Here's the drawing with two shaded views (mm, measured from the low corner). I have some questions. Give positions to 0.01 mm unless a question says otherwise; leave off trailing zeros. Write each loop counter-clockwise with the first axis right and the second up, starting at its lowest first coordinate (ties: lowest second). Pieces come first, ordered by that corner, then holes. Notation, with made-up numbers: (88, -32.75) -> (94, -32.75) arc R19 cw to (94, -22.75) -> close; hole circle Ø9 at (1.5, -38.5). An arc over 180 degrees is marked (long way). One line per item, written item: value.
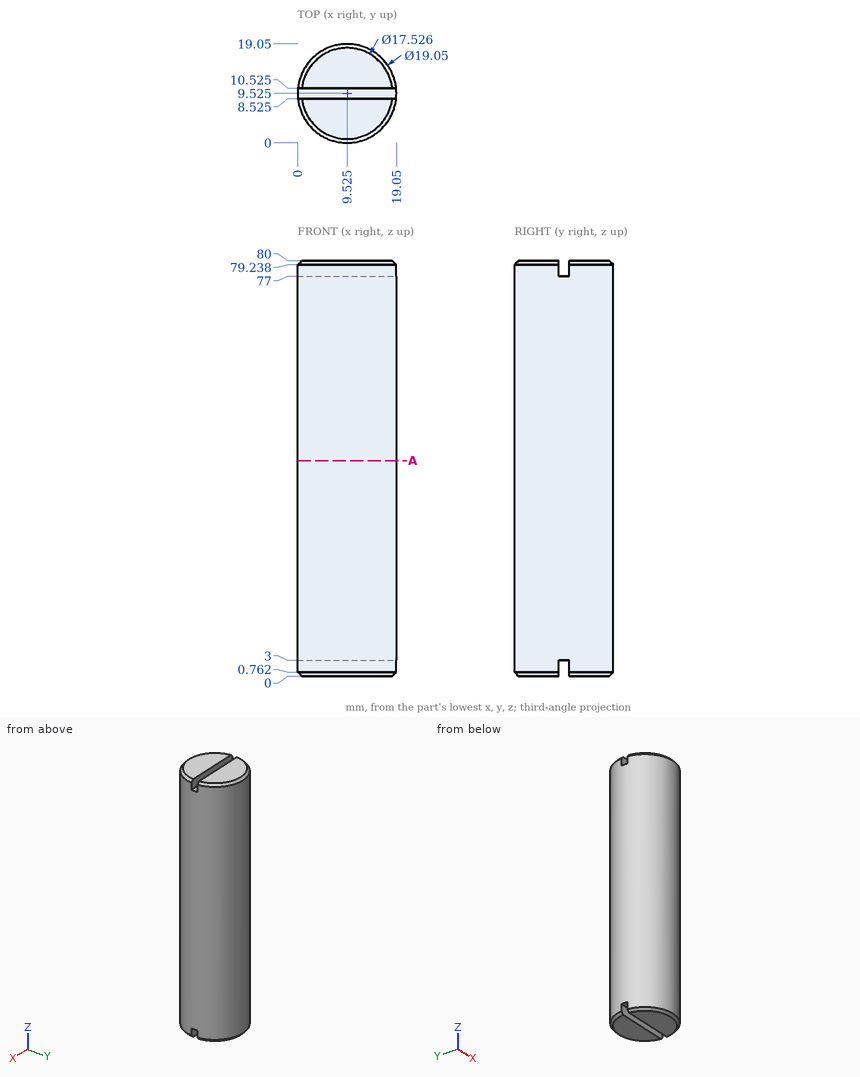
1) If we section it at A-A (z = 41.5): Write out the boundary of the cut face in (x, y) (3 decimals), and give its area (3 significant figures).
Answer list:
outline: circle Ø19.05 at (9.525, 9.525)
area: 285 mm^2
2) I need wall thicknesses on L1, parallel to Y at x = 9.75, z = 49; L2, parallel to X at y = 8.5, z = 55.5; L3, parallel to Z at x = 17.25, y = 9.5. Which ranges of each line are inside material? Lowest first, please.
Answer list:
L1: y = 0 to 19.05
L2: x = 0.06 to 18.99
L3: z = 3 to 77
3) Will these pins go through, and if not, where does the flat tip stop? pin 1 (1 mm diameter, centred on x = 2.5, y = 3, fed in from -Z); pin 2 (2.5 mm diameter, centred on x = 11, z = 79, fed in from -Y); pin 3 (1.5 mm diameter, centred on x = 5.5, z = 1.5, fed in from +Y).
Answer list:
pin 1: stops at z = 0.32
pin 2: stops at y = 0
pin 3: stops at y = 18.47
